Geometry: see drawing. Coordinates: mm, zero at the bounding-box minimum. A direction names the side the tool comes from. Round coordinates to 2 decimals unless told otherwise and drop trailing zeros. Loops run counter-clockwise (first coordinate to the right, second up) from the corner with the lowest first, then second, coordinate; pieces in that order, holes last. Notation, with made-up numbers: M -16.5,3 L 18.5,3 A27 cw 18.5,38 Z; hole C 12,60 d9. An arc over 180 degrees is marked long. Answer as a JSON object with one key per item and string values.
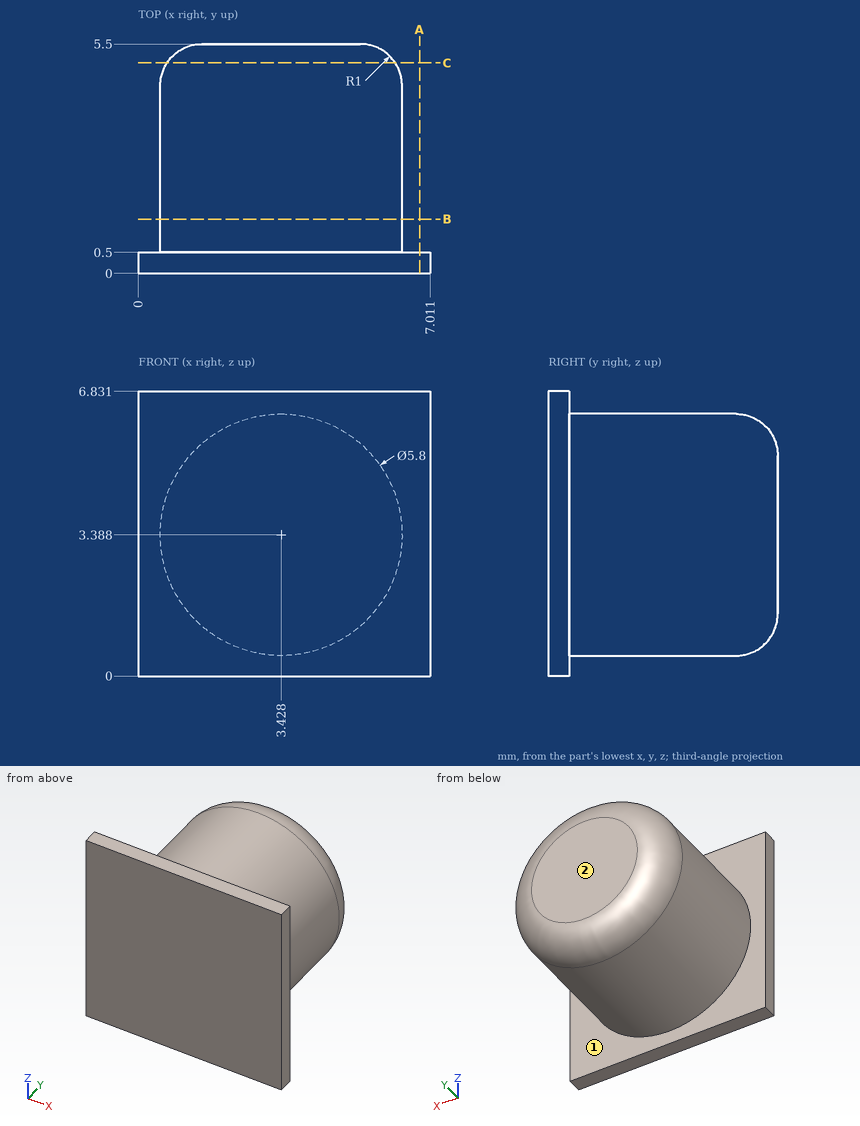
1) Section query B-B (y = 1.3). Return the cut outline in (x, z), and give its area (3 significant figures).
Results:
{"outline": "C 3.43,3.39 d5.8", "area": "26.4 mm2"}
2) Pin query (flat end, axial travel): P1, Ø1.5, axis at x = 6, y = 5, coming from the -Z side; P2, Ø1.5, axis at y = 3, z = 2, coming from the +X side. Return the tip coordinate at first contact, or that it passes through.
Results:
{"P1": "z = 1.21", "P2": "x = 6.26"}
3) Reachability of the marked faces 1 and 2 from +Z, -Z, +X, -X, +Y, -Y: full face, straight path, thin tool, end or side. Return the list, or none.
Results:
{"face 1": "+Y", "face 2": "+Z, -Z, +X, -X, +Y"}
4) Section query A-A (x = 6.75). Return the cut outline in (y, z).
Results:
{"outline": "M 0,0 L 0.5,0 L 0.5,6.83 L 0,6.83 Z"}
5) Ray query, line 1 (Y direction, x = 1, z = 1.25); line 2 (X direction, y = 3.35, z = 1) (1 decimal); line 3 (X direction, y = 2.55, z = 1.75) (1 decimal). Return the intervals inside material, ascending.
Results:
{"line 1": "0 to 0.5", "line 2": "1.8 to 5.1", "line 3": "1 to 5.8"}
6) Section query C-C (y = 5.05). Return the cut outline in (x, z) (1 decimal).
Results:
{"outline": "C 3.4,3.4 d5.5"}
